```python
from build123d import *

# Parameters (mm, degrees)
BOSS_EXTRU_1_DEPTH = 12
ESQUISSE3_W        = 15
ESQUISSE3_H        = 32
BOSS_EXTRU_2_DEPTH = 2
CONG_2_R           = 2
CONG_3_R           = 5


with BuildPart() as part:
    # Esquisse2 → Boss.-Extru.1 (new body)
    with BuildSketch(Plane.XY):
        Polygon((-2.5, -20), (0, -17.5), (0, -10.428932188), (-6.035533906, -16.464466094), align=None)
        Polygon((7.5, -10), (7.5, 0), (0, 0), (0, -10.428932188), (0, -17.5), align=None)
        Polygon((15, 0), (7.5, 0), (7.5, -10), (15, -17.5), (15, -10.428932188), align=None)
        Polygon((15, -10.428932188), (15, -17.5), (17.5, -20), (21.035533906, -16.464466094), align=None)
        Polygon((-3.914213562, -21.414213562), (-7.449747468, -17.878679656), (-6.035533906, -16.464466094), (-2.5, -20), align=None)
        Polygon((17.5, -20), (18.914213562, -21.414213562), (22.449747468, -17.878679656), (21.035533906, -16.464466094), align=None)
    extrude(amount=BOSS_EXTRU_1_DEPTH)

    # Esquisse3 → Boss.-Extru.2 (add)
    with BuildSketch(Plane(origin=(0, 0, 0), x_dir=(1, 0, 0), z_dir=(0, 1, 0))):
        with Locations((7.5, -16)):
            Rectangle(ESQUISSE3_W, ESQUISSE3_H)
    extrude(amount=BOSS_EXTRU_2_DEPTH)

    # Congé2
    cong_2_edges = [part.edges().sort_by_distance(p)[0] for p in [
        (0, -10.428932188, 6),
        (15, -10.428932188, 6),
    ]]
    fillet(cong_2_edges, radius=CONG_2_R)

    # Congé3
    cong_3_edges = [part.edges().sort_by_distance(p)[0] for p in [
        (7.5, 0, 12),
    ]]
    fillet(cong_3_edges, radius=CONG_3_R)


solid = part.part
```
Source: CAD feature listing. Evaluate the final solid. Frame: model axes, mm. A direction names the side the tool comes from. Coordinates: 2 decimals unless noted, no trailing zeros. Loops run counter-clockwise (first coordinate to the right, second up) from the corner with the lowest first, then second, coordinate; pieces in that order, holes last. Notation, with made-up numbers: M 13.25,4 L 56.25,4 A6 cw 56.25,8 Z; hole C 60,15.5 d7. An arc over 180 degrees is marked long. Put each result on its own line as item: value. Start each with the question number.
1) Cut plane D-D on y = -19. Return the cut outline in (x, z).
2) Ray query, L1, parallel to X at y = -19, z = 6; L2, parallel to Z at x = 17, y = -18.5; L3, parallel to X at y = 1, z = 5. Return the intervals inside material, ascending. Write a range as from..to.
3) Cut plane A-A on y = -16. Return the cut outline in (x, z), then the cut area to 3 significant figures.
4) Cut plane B-B on x = 14. Return the cut outline in (y, z), then the cut area to 3 significant figures.
5) Contact query for flat-ended pins moving along their axis: pin 1 Ø2 at (y, z) = (-13, 14) entering from +X; pin 2 Ø5 at (y, z) = (-2, 16.5) entering from +X; pin 3 Ø10 at (x, y) = (4.5, -17.5) entering from +Z; pin 4 Ø12 at (y, z) = (-8.5, 14.5) entering from -X. Output: stop coordinate, or through.
6) Reachability of faces 5 (the face through (0, -3, 9)), 6 (the face through (15, -3, 9)), 7 (the face through (7, -9, 12)), 8 (the face through (20.66, -19.67, 5.92)) from +Z, -Z, +X, -X, +Y, -Y: full face, straight path, thin tool, end or side. Return the list, or none.
7) Pull-direction query (X, two-part tool) for faces 1 (the face through (13.1, -15.6, 5.9)), 2 (the face through (-5.66, -19.67, 5.92)), 3 (the face through (7, -7, 0)), 4 (the face through (1.7, -15.8, 5.9)); classes: pulls with the +X half, pulls with the -X half, needs draft (parallel to the pull), parting line crosses it, or undercut.
8) Cut plane C-C on z = 8. Return the cut outline in (x, y).
The answers:
1. outline: M -6.33,0 L -1.5,0 L -1.5,12 L -6.33,12 Z; M 16.5,0 L 21.33,0 L 21.33,12 L 16.5,12 Z
2. L1: x = -6.33..-1.5, 16.5..21.33
2. L2: z = 0..12
2. L3: x = 0..15
3. outline: M -5.57,0 L 1.5,0 L 1.5,12 L -5.57,12 Z; M 13.5,0 L 20.57,0 L 20.57,12 L 13.5,12 Z
3. area: 170 mm²
4. outline: M -16.5,0 L 2,0 L 2,32 L 0,32 L 0,17 A5 cw -5,12 L -16.5,12 Z
4. area: 267 mm²
5. pin 1: passes through
5. pin 2: stops at x = 15
5. pin 3: stops at z = 12
5. pin 4: stops at x = -3.53
6. face 5: +Z, -Z, -X, +Y
6. face 6: +Z, -Z, +X, +Y
6. face 7: +Z, +X, -X, -Y
6. face 8: +Z, -Z, +X, -Y
7. face 1: undercut
7. face 2: pulls with the -X half
7. face 3: needs draft
7. face 4: undercut
8. outline: M -7.45,-17.88 L -3.91,-21.41 L 7.5,-10 L 18.91,-21.41 L 22.45,-17.88 L 15.59,-11.01 A2 cw 15,-9.6 L 15,2 L 0,2 L 0,-9.6 A2 cw -0.59,-11.01 Z
